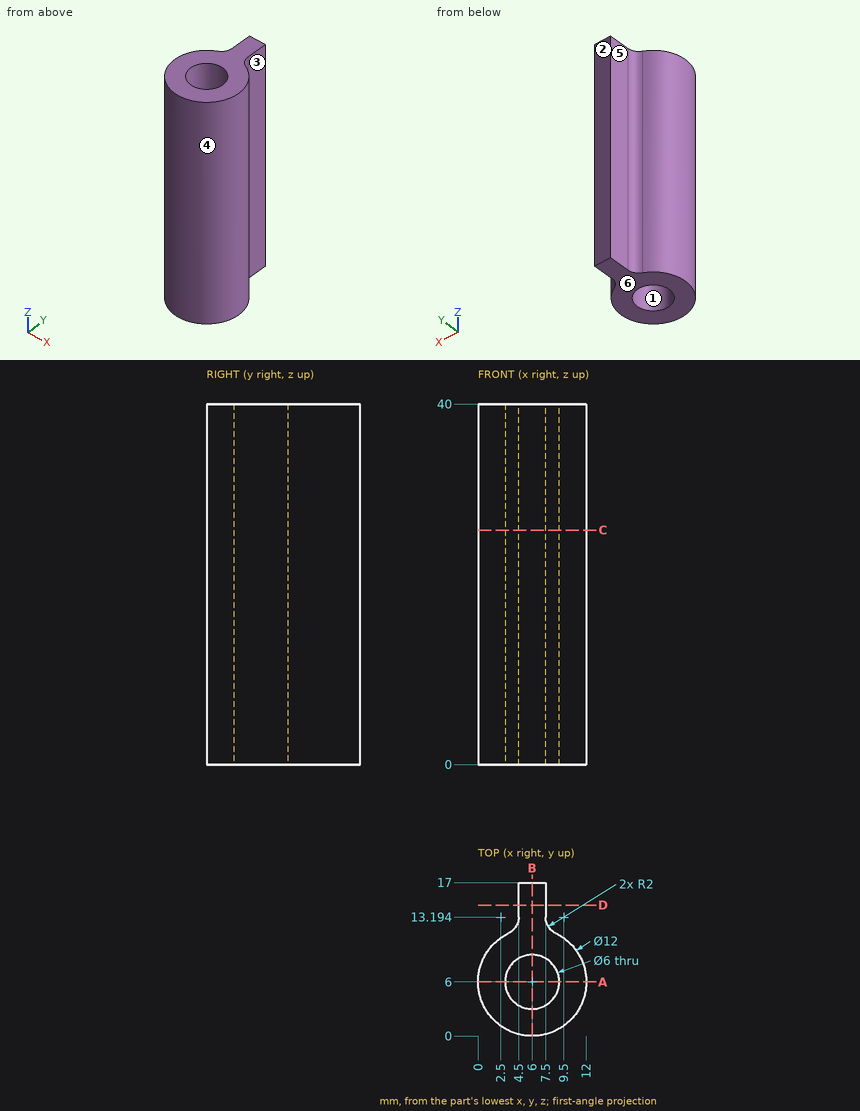
Could you check a few things on this drawing? It's one solid part, dimensions in mm from its lowest x, y, z. A direction names the side the tool comes from. Coordinates: 2 decimals unless noted, no trailing zeros. Order: outer loops, then holes, each group sorted by start corner. A loop starts at its lowest first (then second) coordinate and runs counter-clockwise, first axis right, second up. Notation, with made-up numbers: (80, 69.5) -> (114, 69.5) arc R19 cw to (114, 76.5) -> close; hole circle Ø1 at (8, 0). An arc over 180 degrees is marked (long way). Answer in a Markdown table with one row per item.
(1) I want a section at C-C on z = 26. List the corners of the cut face in (x, y) for me (1 decimal).
Answer key:
| item | result |
|---|---|
| outline | (3.4, 11.4) arc R6 ccw (long way) to (8.6, 11.4) arc R2 cw to (7.5, 13.2) -> (7.5, 17) -> (4.5, 17) -> (4.5, 13.2) arc R2 cw to start; hole circle Ø6 at (6, 6) |
(2) Thinking about a two-plate mould opening in Y: for the marked faces 1, 2, 3 and 4, which applies, +Y half, -Y half, draft (parallel to the pull), parting line (faces both ways), or undercut?
Answer key:
| item | result |
|---|---|
| face 1 | undercut |
| face 2 | +Y half |
| face 3 | draft |
| face 4 | parting line |
(3) I want a section at A-A on y = 6. List the corners of the cut face in (x, z) for me.
Answer key:
| item | result |
|---|---|
| outline | (0, 0) -> (3, 0) -> (3, 40) -> (0, 40) -> close; (9, 0) -> (12, 0) -> (12, 40) -> (9, 40) -> close |
(4) I want a section at D-D on y = 14.5. List the corners of the cut face in (x, z) for me, then the cut area to 3 significant figures.
Answer key:
| item | result |
|---|---|
| outline | (4.5, 0) -> (7.5, 0) -> (7.5, 40) -> (4.5, 40) -> close |
| area | 120 mm^2 |
(5) On a 3-axis mill with a long thin cutter (end or side, diameter ignored), from which of +Z, -Z, +X, -X, +Y, -Y can I reach the whole of each face in a straight line? I mean the marked faces 5 and 6. Say none if no direction works.
Answer key:
| item | result |
|---|---|
| face 5 | +Z, -Z, -X, +Y |
| face 6 | -Z, +X, -X, +Y, -Y |
(6) Will these pins go through, and if not, where does the flat tip stop? pin 1 Ø1.9 at (y, z) = (15.5, 13) entering from +X; pin 2 Ø8 at (y, z) = (14, 18) entering from -X; pin 3 Ø3 at (y, z) = (16, 12) entering from -X.
Answer key:
| item | result |
|---|---|
| pin 1 | x = 7.5 |
| pin 2 | x = 1.53 |
| pin 3 | x = 4.5 |
(7) I want a section at B-B on x = 6. List the corners of the cut face in (y, z) for me.
Answer key:
| item | result |
|---|---|
| outline | (0, 0) -> (3, 0) -> (3, 40) -> (0, 40) -> close; (9, 0) -> (17, 0) -> (17, 40) -> (9, 40) -> close |
(8) Please list where these lines run through material, in increasing order: probe 1 along Y at (x, z) = (6, 17); probe 2 along X at (y, z) = (15, 25.5); probe 3 along X at (y, z) = (7.25, 20).
Answer key:
| item | result |
|---|---|
| probe 1 | 0 to 3, 9 to 17 |
| probe 2 | 4.5 to 7.5 |
| probe 3 | 0.13 to 3.27, 8.73 to 11.87 |
